from build123d import *

# Parameters (mm, degrees)
F0_R     = 11.43
F1_DEPTH = 1.5875
F2_R     = 5.08
F3_DEPTH = 1.27
F4_R     = 4.0005
F5_DEPTH = 3.175
F6_R     = 0.674531


with BuildPart() as f1:
    # F0 (on Top) → F1 (new body)
    with BuildSketch(Plane.XY):
        Circle(F0_R)
    extrude(amount=F1_DEPTH)

    # F2 (on face) → F3 (join)
    with BuildSketch(Plane.XY.offset(1.5875)):
        Circle(F2_R)
    extrude(amount=F3_DEPTH)

    # F4 (on face) → F5 (join)
    with BuildSketch(Plane.XY.offset(2.8575)):
        Circle(F4_R)
    extrude(amount=F5_DEPTH)

    # F6
    f6_edges = [f1.edges().sort_by_distance(p)[0] for p in [
        (-11.43, 0, 0),
    ]]
    fillet(f6_edges, radius=F6_R)


solid = f1.part
Design review of the part built by this model. Coordinates are the model's own, in mm. A direction names the side the tool comes from. Round coordinates to 2 decimals unless told otherwise and drop trailing zeros. Loops run counter-clockwise (first coordinate to the right, second up) from the corner with the lowest first, then second, coordinate; pieces in that order, holes last. Notation, with made-up numbers: (47.5, 6) - (51.5, 6) arc R34 ccw to (51.5, 45) - close; hole circle Ø11 at (-28.5, 58). An arc over 180 degrees is marked (long way). One line per question, with ' | ' between items.
1. We need section A-A, the plane y = 0. State the section outline as (x, z) points, and give its area (3 significant figures).
Results are:
outline: (-11.43, 0.67) arc R0.67 ccw to (-10.76, 0) - (10.76, 0) arc R0.67 ccw to (11.43, 0.67) - (11.43, 1.59) - (5.08, 1.59) - (5.08, 2.86) - (4, 2.86) - (4, 6.03) - (-4, 6.03) - (-4, 2.86) - (-5.08, 2.86) - (-5.08, 1.59) - (-11.43, 1.59) - close | area: 74.4 mm²
2. Clearance check with flat-ended pins moving along their axes: P1, Ø1.5, axis at x = -4, z = 2, coming from the -Y side; P2, Ø6, axis at x = -4.5, y = 4, coming from the +Z side; P3, Ø4, axis at x = 9, y = 6.5, coming from the +Z side. State where each tip first meets the part, or that it passes through.
Results are:
P1: stops at y = -10.92 | P2: stops at z = 6.03 | P3: stops at z = 1.59
3. For L1, parallel to Z at x = 9.75, y = 4.25; L2, parallel to Y at x = 3, z = 3.75; L3, parallel to X at y = 2.5, z = 0.75, list the stretches that pass through material, from the lowest coordinate up. Write a range as [from, to].
Results are:
L1: z = [0, 1.59] | L2: y = [-2.65, 2.65] | L3: x = [-11.15, 11.15]
4. For faces 1 (the face through (10.902, 3.433, 1.125)), 2 (the face through (-0.9, -3.9, 4.4)), list the 3-axis set-ups (+Z, -Z, +X, -X, +Y, -Y) from which the entire face can be reached by the end or side of a thin tool; tool diameter is ignored.
Results are:
face 1: +Z, -Z | face 2: +Z
5. We need section C-C, the plane z = 5. State the section outline as (x, y) points, and give its area (3 significant figures).
Results are:
outline: circle Ø8 at (0, 0) | area: 50.3 mm²
